Read the model definition and answer for the solid it produces. Units are mm, in the model's axes. Give positions to 0.01 mm unless a question says otherwise; leave off trailing zeros. Order: outer loops, then holes, each group sorted by start corner. A loop starts at its lowest first (then second) coordinate and runs counter-clockwise, first axis right, second up. Notation, with made-up numbers: M 83.25,43.5 L 100.25,43.5 A30 ccw 100.25,68.5 Z; hole C -17.75,38.25 d11. An arc over 180 degrees is marked long. One line per item, written item: value. Start each with the question number.
from build123d import *

# Parameters (mm, degrees)
BOSS_EXTRUDE1_DEPTH          = 2.5
F_5_32_0_14_DIAMETER_HOLE1_D = 3.556
LPATTERN1_COUNT              = 7
LPATTERN1_PITCH              = 5
MIRROR1_COPY_1_D             = 3.556
MIRROR1_COPY_2_D             = 3.556
MIRROR1_COPY_3_D             = 3.556
MIRROR1_COPY_4_D             = 3.556
MIRROR1_COPY_5_D             = 3.556
MIRROR1_COPY_6_D             = 3.556
MIRROR1_COPY_7_D             = 3.556


with BuildPart() as part:
    # Sketch1 → Boss-Extrude1 (new body)
    with BuildSketch(Plane(origin=(0, 0, 0), x_dir=(0, 0, -1), z_dir=(1, 0, 0))):
        with BuildLine():
            Line((5, 30), (5, -30))
            ThreePointArc((5, -30), (0, -35), (-5, -30))
            Line((-5, -30), (-5, 30))
            ThreePointArc((-5, 30), (0, 35), (5, 30))
        make_face()
    extrude(amount=BOSS_EXTRUDE1_DEPTH)

    # 5/32 (0.14) Diameter Hole1 (through all)
    with Locations(Plane(origin=(2.5, 0, 0), x_dir=(0, 0, -1), z_dir=(1, 0, 0))):
        with Locations((0, 0)):
            f_5_32_0_14_diameter_hole1 = Hole(F_5_32_0_14_DIAMETER_HOLE1_D / 2)

    # LPattern1: 5/32 (0.14) Diameter Hole1 ×7
    with Locations(*[(0, i * LPATTERN1_PITCH, 0) for i in range(1, LPATTERN1_COUNT)]):
        add(f_5_32_0_14_diameter_hole1, mode=Mode.SUBTRACT)

    # Mirror1 copy 1 (through all)
    with Locations(Plane(origin=(2.5, -5, 0), x_dir=(0, 0, -1), z_dir=(1, 0, 0))):
        with Locations((0, 0)):
            Hole(MIRROR1_COPY_1_D / 2)

    # Mirror1 copy 2 (through all)
    with Locations(Plane(origin=(2.5, -10, 0), x_dir=(0, 0, -1), z_dir=(1, 0, 0))):
        with Locations((0, 0)):
            Hole(MIRROR1_COPY_2_D / 2)

    # Mirror1 copy 3 (through all)
    with Locations(Plane(origin=(2.5, -15, 0), x_dir=(0, 0, -1), z_dir=(1, 0, 0))):
        with Locations((0, 0)):
            Hole(MIRROR1_COPY_3_D / 2)

    # Mirror1 copy 4 (through all)
    with Locations(Plane(origin=(2.5, -20, 0), x_dir=(0, 0, -1), z_dir=(1, 0, 0))):
        with Locations((0, 0)):
            Hole(MIRROR1_COPY_4_D / 2)

    # Mirror1 copy 5 (through all)
    with Locations(Plane(origin=(2.5, -25, 0), x_dir=(0, 0, -1), z_dir=(1, 0, 0))):
        with Locations((0, 0)):
            Hole(MIRROR1_COPY_5_D / 2)

    # Mirror1 copy 6 (through all)
    with Locations(Plane(origin=(2.5, -30, 0), x_dir=(0, 0, -1), z_dir=(1, 0, 0))):
        with Locations((0, 0)):
            Hole(MIRROR1_COPY_6_D / 2)

    # Mirror1 copy 7 (through all)
    with Locations(Plane(origin=(2.5, 0, 0), x_dir=(0, 0, -1), z_dir=(1, 0, 0))):
        with Locations((0, 0)):
            Hole(MIRROR1_COPY_7_D / 2)


solid = part.part
Q1. Determine the mould class of faces 1 (the flat face through (1, 0, -5)), 2 (the cylindrical face through (1.233, 26.763, -0.231)), 3 (the flat face through (2.5, 0, -2)) for opening direction Z: released by +Z, released by -Z, zero draft, split by the parting line, or undercut.
Q2. Consider probe 1 along Z at (x, y) = (1.7, -9); probe 2 along Z at (x, y) = (2, 19.5); probe 3 along Y at (x, z) = (0.3, -4). Determine where each line is inside the solid, lowest interval first.
Q3. Find section B-B, the plane x = 2.1. State how many separate pieces and enclosed holes the cut face has, then the cut area to 3 significant figures.
Q4. Find section A-A, the plane y = 5. Give the vertices of the cut face in (x, z).
Q5. Find section D-D, the plane z = 3. Give the vertices of the cut face in (x, y).
Q6. Each of these flat-tipped pins is pushed along its axis until it touches: pin 1 (2 mm diameter, centred on y = 30, z = 0, fed in from +X); pin 2 (1 mm diameter, centred on x = 1.5, z = -4, fed in from +Y). Where does it stop, or does it pass through?
Evaluation:
1. face 1: released by -Z
1. face 2: undercut
1. face 3: zero draft
2. probe 1: -5 to -1.47, 1.47 to 5
2. probe 2: -5 to -1.71, 1.71 to 5
2. probe 3: -33 to 33
3. separate pieces: 1
3. enclosed holes: 13
3. area: 549 mm2
4. outline: M 0,-5 L 2.5,-5 L 2.5,-1.78 L 0,-1.78 Z; M 0,1.78 L 2.5,1.78 L 2.5,5 L 0,5 Z
5. outline: M 0,-34 L 2.5,-34 L 2.5,34 L 0,34 Z
6. pin 1: through
6. pin 2: y = 33.57
